Here's the drawing with two shaded views (mm, measured from the low corner). I have some questions. A direction names the side the tool comes from. Coordinates: 2 decimals unless noted, no trailing zeros. Loops run counter-clockwise (first coordinate to the right, second up) from the corner with the lowest first, then second, coordinate; pieces in that order, holes last. Notation, with made-up numbers: M 72.5,8.25 L 98.5,8.25 A11 cw 98.5,23.25 Z; hole C 68,-40 d3. An arc over 180 degrees is marked long. Return JSON: item names as keys, results as strings. Group by question number.
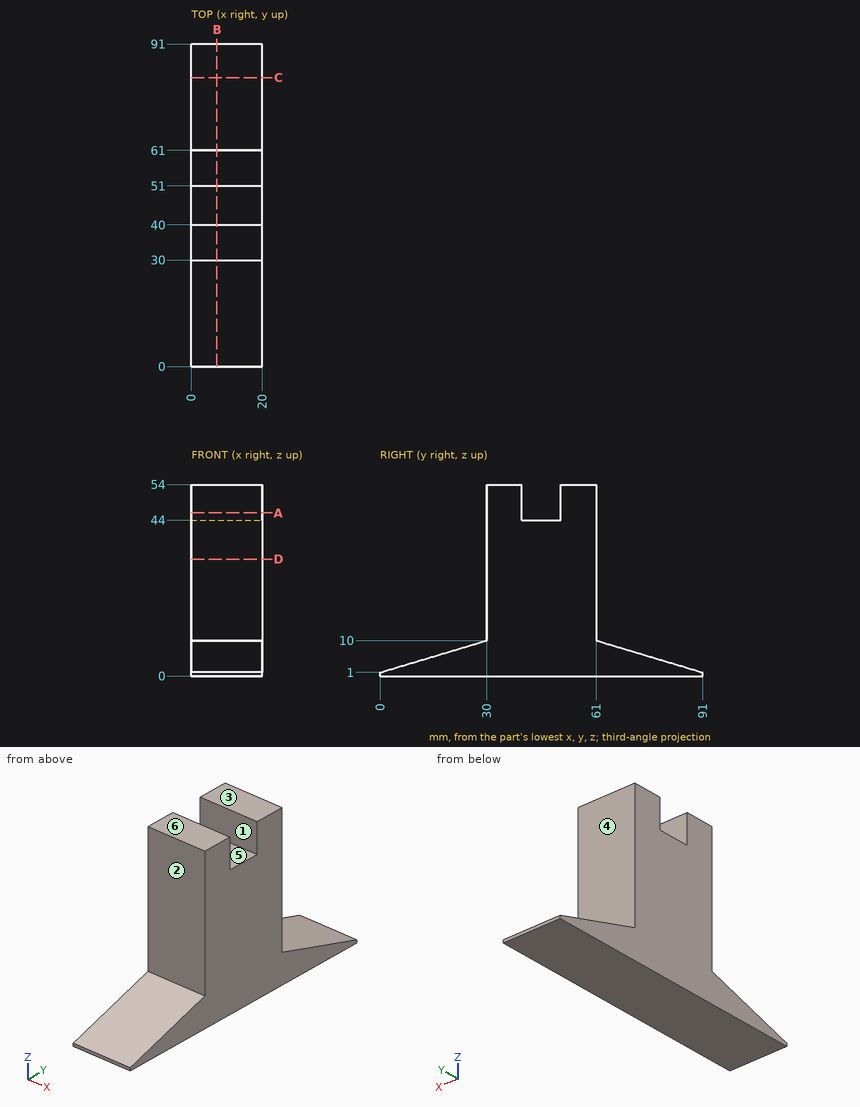
(1) Imagine slicing it at C-C, the plane y = 81.5. Write out the boundary of the cut face in (x, z).
(2) Imagine slicing it at B-B, the plane x = 7.25. Write out the boundary of the cut face in (y, z).
(3) Imagine slicing it at D-D, the plane z = 33. Write out the boundary of the cut face in (x, y).
(4) Will these pins go through, and if not, where does the flat tip stop? P1, Ø12, axis at x = 16.5, z = 19.5, coming from the +Y side; P2, Ø8, axis at x = 13.5, z = 46.5, coming from the -Y side.
(5) We'd pull the mould along Y, two halves only. Please class the marked faces 4, 5 and 6: +Y half, -Y half, draft (parallel to the pull), parting line (faces both ways), or undercut.
(6) For the marked faces 1, 2 and 3, which set-ups out of +Z, -Z, +X, -X, +Y, -Y let a thin tool reach every point of the face, with its end or its side?
(7) Imagine slicing it at A-A, the plane z = 46. Write out the boundary of the cut face in (x, y), then the cut area to 3 significant figures.
(8) If I drill on L1, parallel to Y at x = 8.25, z = 44.5; L2, parallel to Y at x = 1, z = 39; L3, parallel to Z at x = 14.75, y = 44.5, over which ranges is the centre line in solid material (lowest first)? Write a range as [from, to].
Checks:
{
 "1": {"outline": "M 0,0 L 20,0 L 20,3.85 L 0,3.85 Z"},
 "2": {"outline": "M 0,0 L 91,0 L 91,1 L 61,10 L 61,54 L 51,54 L 51,44 L 40,44 L 40,54 L 30,54 L 30,10 L 0,1 Z"},
 "3": {"outline": "M 0,30 L 20,30 L 20,61 L 0,61 Z"},
 "4": {"P1": "y = 61", "P2": "y = 30"},
 "5": {"face 4": "+Y half", "face 5": "undercut", "face 6": "draft"},
 "6": {"face 1": "+Z, +X, -X", "face 2": "+Z, +X, -X, -Y", "face 3": "+Z, +X, -X, +Y, -Y"},
 "7": {"outline": "M 0,30 L 20,30 L 20,40 L 0,40 Z; M 0,51 L 20,51 L 20,61 L 0,61 Z", "area": "400 mm²"},
 "8": {"L1": "[30, 40], [51, 61]", "L2": "[30, 61]", "L3": "[0, 44]"}
}
